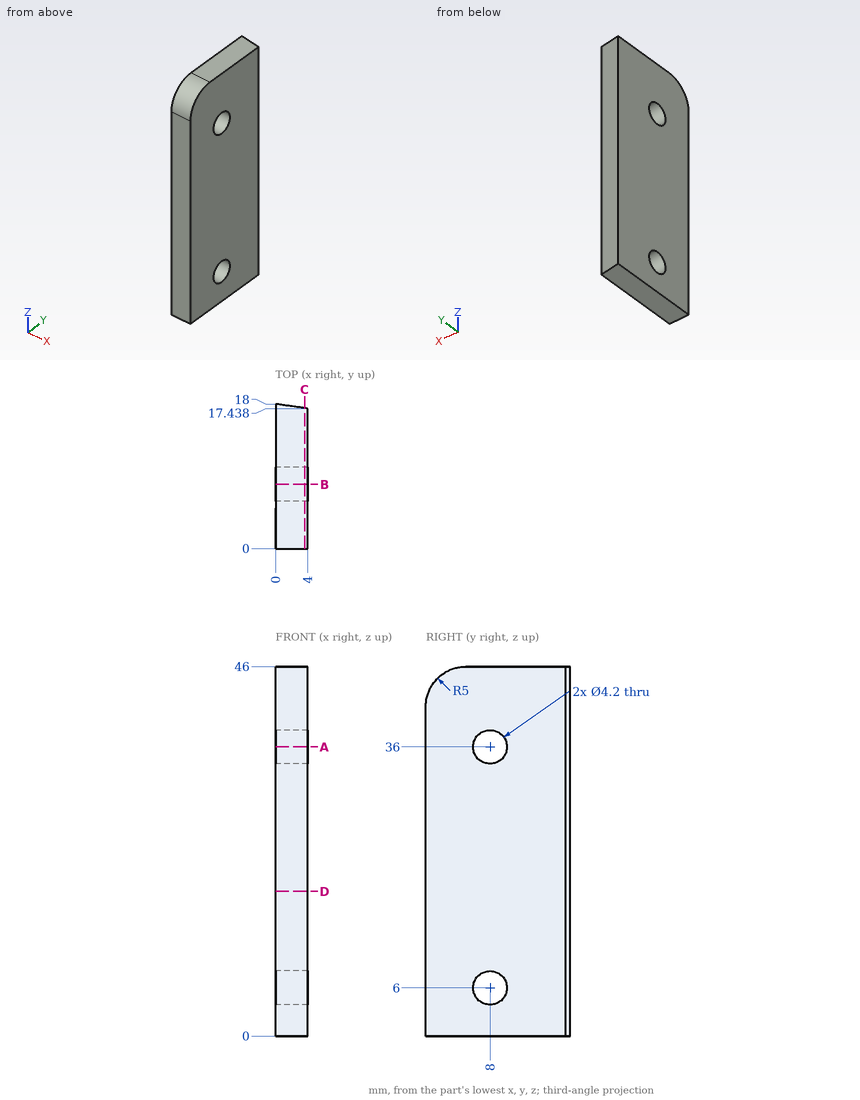
Input: dimensioned drawing with shaded views. Units: mm. Origin: part minimum x, y, z. Give positions to 0.01 mm unless a question says otherwise; leave off trailing zeros. Order: outer loops, then holes, each group sorted by start corner. A loop starts at its lowest first (then second) coordinate and runs counter-clockwise, first axis right, second up.
(1) Section query D-D (z = 18). Return the cut outline in (x, y).
(2) Section query C-C (x = 3.6). Return the cut outline in (y, z), plus the area to 3 significant figures.
(3) Section query B-B (y = 8). Return the cut outline in (x, z), plus the area to 3 significant figures.
(4) Material intervals for line 1 along Z through (x, y) = (2.15, 7.25); line 2 along Y through (x, z) = (1.9, 6); line 3 along Z through (x, y) = (2.6, 9), sorted ascending.
(5) Section query A-A (z = 36). Return the cut outline in (x, y), plus the area to 3 significant figures.
(6) Contact query for flat-ended pins moving along their axis: P1, Ø4, axis at y = 8, z = 6, coming from the +X side; P2, Ø5, axis at y = 8, z = 36, coming from the +X side. Output: stop coordinate, or through.
Outcome:
1. outline: (0, 0) - (4, 0) - (4, 17.44) - (0, 18) - close
2. outline: (0, 0) - (17.49, 0) - (17.49, 46) - (5, 46) arc R5 ccw to (0, 41) - close; hole circle Ø4.2 at (8, 6); hole circle Ø4.2 at (8, 36)
2. area: 772 mm2
3. outline: (0, 0) - (4, 0) - (4, 3.9) - (0, 3.9) - close; (0, 8.1) - (4, 8.1) - (4, 33.9) - (0, 33.9) - close; (0, 38.1) - (4, 38.1) - (4, 46) - (0, 46) - close
3. area: 150 mm2
4. line 1: z = 0 to 4.04, 7.96 to 34.04, 37.96 to 46
4. line 2: y = 0 to 5.9, 10.1 to 17.73
4. line 3: z = 0 to 4.15, 7.85 to 34.15, 37.85 to 46
5. outline: (0, 0) - (4, 0) - (4, 5.9) - (0, 5.9) - close; (0, 10.1) - (4, 10.1) - (4, 17.44) - (0, 18) - close
5. area: 54.1 mm2
6. P1: passes through
6. P2: stops at x = 4
